Geometry check sheet. Reference: drawing and pictorial views, mm from the part's lowest x, y, z. Round coordinates to 2 decimals unless told otherwise and drop trailing zeros. Order: outer loops, then holes, each group sorted by start corner. A loop starts at its lowest first (then second) coordinate and runs counter-clockwise, first axis right, second up. Notation, with made-up numbers: (-23.75, -2) -> (-15.75, -2) arc R35 cw to (-15.75, 33) -> close; hole circle Ø11 at (46.25, 16). An arc over 180 degrees is marked (long way). Put each result on its own line as item: value.
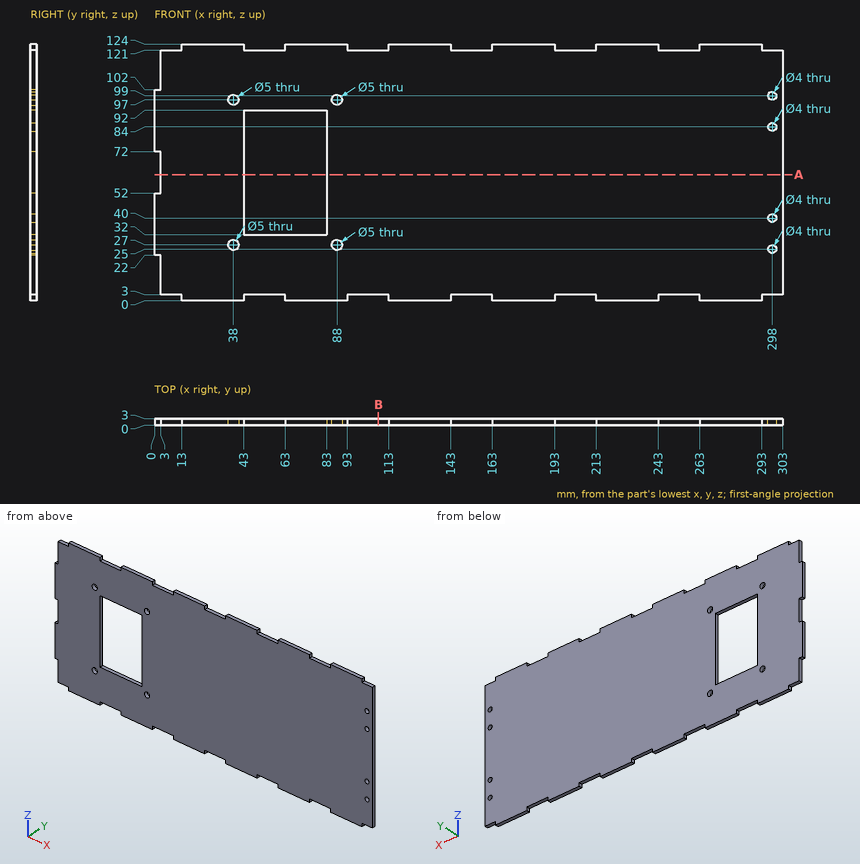
Item 1: Depth check by flat-ended pin: pin 1 Ø1.5 at (y, z) = (1, 123) entering from +X; pin 2 Ø1.5 at (x, y) = (100.5, 0.5) entering from +Z; pin 3 Ø0.9 at (y, z) = (1.5, 1) entering from -X; pin 4 Ø3 at (x, z) = (298, 25) entering from +Y. Enter the tip coordinate at first touch or a pass-through.
Geometry check:
pin 1: x = 293
pin 2: z = 121
pin 3: x = 13
pin 4: through
Item 2: Sectioned sample at A-A, the plane z = 61. Record the boundary of the cut face in (x, y).
Geometry check:
outline: (3, 0) -> (43, 0) -> (43, 3) -> (3, 3) -> close; (83, 0) -> (303, 0) -> (303, 3) -> (83, 3) -> close
Item 3: Sectioned sample at B-B, the plane x = 108. Record the boundary of the cut face in (y, z), then the cut area to 3 significant figures.
Geometry check:
outline: (0, 3) -> (3, 3) -> (3, 121) -> (0, 121) -> close
area: 354 mm2
Item 4: Material ranges on line 1 along Z through (x, y) = (88, 0.9); line 2 along X through (y, z) = (2.1, 84); line 3 along Z through (x, y) = (298, 1.3), recorded low to high.
Geometry check:
line 1: 0 to 24.5, 29.5 to 94.5, 99.5 to 124
line 2: 0 to 43, 83 to 296, 300 to 303
line 3: 3 to 23, 27 to 38, 42 to 82, 86 to 97, 101 to 121
